Geometry: final body of the model. Coordinates: model frame, mm. A direction names the side the tool comes from. Give positions to 0.01 mm unless a question says otherwise; leave off trailing zeros. Order: outer loops, then holes, each group sorted by start corner. A loop starts at its lowest first (then second) coordinate and runs counter-clockwise, first axis right, second up. Notation, with made-up numbers: (26, 36.5) -> (45, 36.5) arc R34 cw to (45, 74.5) -> close; hole circle Ø6 at (-36.5, 16). An arc over 180 degrees is marked (long way). One line per question, with ' | ' between items. Start each with the question number.
(1) Set-up query: faces 1 (the face through (-11, 17.75, -5)), 2 (the face through (10.5, 0, 0)), 3 (the face through (-12, 0, 0)). Return all of +Z, -Z, +X, -X, +Y, -Y with unobstructed straight access to the full face (end or side cutting, diameter ignored); none if empty.
(2) First-contact query: pin 1 Ø2.5 at (x, z) = (-10.5, -1) entering from -Y; pin 2 Ø0.5 at (x, z) = (11.5, 5) entering from +Y; pin 3 Ø8 at (x, z) = (-3.5, 4) entering from +Y; pin 4 Ø1.2 at (x, y) = (11.5, 16) entering from +Z. Flat tips, straight axial feed; report the tip coordinate or a pass-through.
(3) Section D-D (y = 13.5). Return loops of the section in (x, z), then the cut area to 4 significant figures.
(4) Mould query, pull axis Z, two halves, no side actions, for faces 4 (the face through (11.49, 0.3, -9.76)), 5 (the face through (-11, -17.75, -5)), 6 (the face through (0, 0, 10.25)). Classes: +Z half, -Z half, draft (parallel to the pull), parting line (faces both ways), or undercut.
(5) Section B-B (z = -4). Return loops of the section in (x, y).
(6) Section C-C (x = -1.25). Return loops of the section in (y, z), then the cut area to 3 significant figures.
(7) Ray query, L1, parallel to Z at x = -1.5, y = 4; L2, parallel to X at y = 9.5, z = 7.5; L3, parallel to Z at x = 10.25, y = -3.5. Return the intervals inside material, ascending.
(8) Section A-A (z = -1.75). Return loops of the section in (x, y).
```python
from build123d import *

# Parameters (mm, degrees)
SKETCH2_W                       = 20.999999999999993
SKETCH2_H                       = 18.500000000000007
BOSS_EXTRUDE2_DEPTH             = 20.5
BOSS_EXTRUDE5_REACH             = 27.871
BOSS_EXTRUDE5_DIRECTION_2_REACH = 27.871
CUT_EXTRUDE1_DEPTH              = 34.81290434139014
CHAMFER1_SIZE                   = 1
CHAMFER1_OF_MIRROR1_SIZE        = 1


with BuildPart() as part:
    # Sketch2 → Boss-Extrude2 (new body)
    with BuildSketch(Plane(origin=(0, 0, 0), x_dir=(1, 0, 0), z_dir=(0, 1, 0))):
        Polygon((-11.999999999999991, -10.249999999999988), (12, -10.249999999999982), (11.999999999999998, 10.249999999999982), (-11.999999999999991, 10.249999999999979), align=None)
        Rectangle(SKETCH2_W, SKETCH2_H, mode=Mode.SUBTRACT)
    boss_extrude2 = extrude(amount=BOSS_EXTRUDE2_DEPTH)

    # Boss-Extrude5: up to this face of the body (flat: up to its plane)
    boss_extrude5_end = Plane(part.part.faces().sort_by_distance((12, 10.25, 0))[0])
    # Sketch4 → Boss-Extrude5 (add, up to the picked face)
    with BuildSketch(Plane(origin=(0, 0, 0), x_dir=(0, 0, -1), z_dir=(1, 0, 0)), mode=Mode.PRIVATE) as boss_extrude5_sk1:
        Polygon((-10.249999999999982, 20.5), (-9.249999999999988, 21.5), (-9.249999999999988, 20.5), align=None)
    boss_extrude5_tool1 = split(extrude(boss_extrude5_sk1.sketch, amount=BOSS_EXTRUDE5_REACH, mode=Mode.PRIVATE), bisect_by=boss_extrude5_end, keep=Keep.BOTH, mode=Mode.PRIVATE)
    # Sketch4 → Boss-Extrude5 (add, up to the picked face)
    with BuildSketch(Plane(origin=(0, 0, 0), x_dir=(0, 0, -1), z_dir=(1, 0, 0)), mode=Mode.PRIVATE) as boss_extrude5_sk2:
        Polygon((10.25, 20.500000000000004), (9.250000000000005, 21.500000000000004), (9.250000000000005, 20.500000000000004), align=None)
    boss_extrude5_tool2 = split(extrude(boss_extrude5_sk2.sketch, amount=BOSS_EXTRUDE5_REACH, mode=Mode.PRIVATE), bisect_by=boss_extrude5_end, keep=Keep.BOTH, mode=Mode.PRIVATE)
    boss_extrude5_1 = boss_extrude5_tool1.solids().sort_by(Axis((0, 20.833333, 9.583333), (1, 0, 0)))[0]
    add(boss_extrude5_1)
    boss_extrude5_2 = boss_extrude5_tool2.solids().sort_by(Axis((0, 20.833333, -9.583333), (1, 0, 0)))[0]
    add(boss_extrude5_2)
    boss_extrude5 = boss_extrude5_1 + boss_extrude5_2  # Boss-Extrude5 as one shape, for the pattern or mirror that repeats it

    # Boss-Extrude5 direction 2: up to this face of the body (flat: up to its plane)
    boss_extrude5_direction_2_end = Plane(part.part.faces().sort_by_distance((-12, 10.25, 0))[0])
    # Sketch4 → Boss-Extrude5 direction 2 (add, up to the picked face)
    with BuildSketch(Plane(origin=(0, 0, 0), x_dir=(0, 0, -1), z_dir=(1, 0, 0)), mode=Mode.PRIVATE) as boss_extrude5_direction_2_sk1:
        Polygon((-10.249999999999982, 20.5), (-9.249999999999988, 21.5), (-9.249999999999988, 20.5), align=None)
    boss_extrude5_direction_2_tool1 = split(extrude(boss_extrude5_direction_2_sk1.sketch, amount=-BOSS_EXTRUDE5_DIRECTION_2_REACH, mode=Mode.PRIVATE), bisect_by=boss_extrude5_direction_2_end, keep=Keep.BOTH, mode=Mode.PRIVATE)
    # Sketch4 → Boss-Extrude5 direction 2 (add, up to the picked face)
    with BuildSketch(Plane(origin=(0, 0, 0), x_dir=(0, 0, -1), z_dir=(1, 0, 0)), mode=Mode.PRIVATE) as boss_extrude5_direction_2_sk2:
        Polygon((10.25, 20.500000000000004), (9.250000000000005, 21.500000000000004), (9.250000000000005, 20.500000000000004), align=None)
    boss_extrude5_direction_2_tool2 = split(extrude(boss_extrude5_direction_2_sk2.sketch, amount=-BOSS_EXTRUDE5_DIRECTION_2_REACH, mode=Mode.PRIVATE), bisect_by=boss_extrude5_direction_2_end, keep=Keep.BOTH, mode=Mode.PRIVATE)
    boss_extrude5_direction_2_1 = boss_extrude5_direction_2_tool1.solids().sort_by(Axis((0, 20.833333, 9.583333), (-1, 0, 0)))[0]
    add(boss_extrude5_direction_2_1)
    boss_extrude5_direction_2_2 = boss_extrude5_direction_2_tool2.solids().sort_by(Axis((0, 20.833333, -9.583333), (-1, 0, 0)))[0]
    add(boss_extrude5_direction_2_2)
    boss_extrude5_direction_2 = boss_extrude5_direction_2_1 + boss_extrude5_direction_2_2  # Boss-Extrude5 direction 2 as one shape, for the pattern or mirror that repeats it

    # Sketch5 → Cut-Extrude1 (cut, through all)
    with BuildSketch(Plane(origin=(11.999999999999998, 0, -1.02e-15), x_dir=(0, 0, -1), z_dir=(1, 0, 0))):
        with BuildLine():
            Line((-6.9999999999999885, 17.750000000000004), (-2.9999999999999893, 17.750000000000004))
            ThreePointArc((-2.9999999999999893, 17.750000000000004), (-2.646446609406713, 17.603553390593277), (-2.4999999999999893, 17.25))
            Line((-2.4999999999999893, 17.25), (-2.4999999999999893, 15.75))
            ThreePointArc((-2.4999999999999893, 15.75), (-2.6464466094067154, 15.396446609406727), (-2.9999999999999893, 15.250000000000002))
            Line((-2.9999999999999893, 15.250000000000002), (-6.9999999999999885, 15.250000000000002))
            ThreePointArc((-6.9999999999999885, 15.250000000000002), (-7.353553390593261, 15.396446609406727), (-7.4999999999999885, 15.75))
            Line((-7.4999999999999885, 15.75), (-7.49999999999999, 17.25))
            ThreePointArc((-7.49999999999999, 17.25), (-7.353553390593265, 17.603553390593277), (-6.9999999999999885, 17.750000000000004))
        make_face()
        with BuildLine():
            Line((7.00000000000001, 17.750000000000004), (3.000000000000011, 17.750000000000004))
            ThreePointArc((3.000000000000011, 17.750000000000004), (2.646446609406735, 17.603553390593277), (2.500000000000011, 17.25))
            Line((2.500000000000011, 17.25), (2.500000000000011, 15.75))
            ThreePointArc((2.500000000000011, 15.75), (2.6464466094067376, 15.396446609406725), (3.000000000000012, 15.250000000000002))
            Line((3.000000000000012, 15.250000000000002), (7.0000000000000115, 15.250000000000004))
            ThreePointArc((7.0000000000000115, 15.250000000000004), (7.353553390593284, 15.39644660940673), (7.500000000000011, 15.750000000000004))
            Line((7.500000000000011, 15.750000000000004), (7.500000000000012, 17.250000000000004))
            ThreePointArc((7.500000000000012, 17.250000000000004), (7.3535533905932855, 17.603553390593277), (7.00000000000001, 17.750000000000004))
        make_face()
    cut_extrude1 = extrude(amount=-CUT_EXTRUDE1_DEPTH, mode=Mode.SUBTRACT)

    # Chamfer1
    chamfer1_edges = [part.edges().sort_by_distance(p)[0] for p in [
        (-11.999999999999991, 10.25, -10.249999999999979),
        (11.999999999999998, 10.25, -10.249999999999982),
        (12, 10.25, 10.249999999999982),
        (-11.999999999999991, 10.25, 10.249999999999988),
        (10.5, 10.25, -9.250000000000018),
        (-10.499999999999991, 10.25, -9.250000000000018),
        (-10.499999999999991, 10.25, 9.249999999999988),
        (10.5, 10.25, 9.249999999999988),
    ]]
    chamfer(chamfer1_edges, length=CHAMFER1_SIZE)


with BuildPart() as mirror1_1:
    # Mirror1: Boss-Extrude2, Boss-Extrude5, Boss-Extrude5 direction 2 across plane
    add(boss_extrude2.mirror(Plane.ZX))
    add(boss_extrude5.mirror(Plane.ZX))
    add(boss_extrude5_direction_2.mirror(Plane.ZX))

    # Mirror1 2: Cut-Extrude1 across plane
    add(cut_extrude1.mirror(Plane.ZX), mode=Mode.SUBTRACT)

    # Chamfer1 of Mirror1
    chamfer1_of_mirror1_edges = [mirror1_1.edges().sort_by_distance(p)[0] for p in [
        (-11.999999999999991, -10.25, -10.249999999999979),
        (11.999999999999998, -10.25, -10.249999999999982),
        (12, -10.25, 10.249999999999982),
        (-11.999999999999991, -10.25, 10.249999999999988),
        (10.5, -10.25, -9.250000000000018),
        (-10.499999999999991, -10.25, -9.250000000000018),
        (-10.499999999999991, -10.25, 9.249999999999988),
        (10.5, -10.25, 9.249999999999988),
    ]]
    chamfer(chamfer1_of_mirror1_edges, length=CHAMFER1_OF_MIRROR1_SIZE)


with BuildPart() as part_1:
    add(part.part)

    # Mirror1 united with what the copies touc: union Mirror1_1
    add(mirror1_1.part)


solid = part_1.part
```
Response:
1) face 1: +X, -X | face 2: +Y, -Y | face 3: +Z, -Z, -X, +Y, -Y
2) pin 1: stops at y = -20.5 | pin 2: stops at y = 20.5 | pin 3: passes through | pin 4: stops at z = 10.25
3) outline: (-12, -9.25) -> (-11, -10.25) -> (11, -10.25) -> (12, -9.25) -> (12, 9.25) -> (11, 10.25) -> (-11, 10.25) -> (-12, 9.25) -> close; hole (-10.5, -8.25) -> (-9.5, -9.25) -> (9.5, -9.25) -> (10.5, -8.25) -> (10.5, 8.25) -> (9.5, 9.25) -> (-9.5, 9.25) -> (-10.5, 8.25) -> close | area: 103.5 mm^2
4) face 4: -Z half | face 5: undercut | face 6: +Z half
5) outline: (-12, -20.5) -> (-10.5, -20.5) -> (-10.5, -17.75) -> (-12, -17.75) -> close; (-12, -15.25) -> (-10.5, -15.25) -> (-10.5, 15.25) -> (-12, 15.25) -> close; (-12, 17.75) -> (-10.5, 17.75) -> (-10.5, 20.5) -> (-12, 20.5) -> close; (10.5, -20.5) -> (12, -20.5) -> (12, -17.75) -> (10.5, -17.75) -> close; (10.5, -15.25) -> (12, -15.25) -> (12, 15.25) -> (10.5, 15.25) -> close; (10.5, 17.75) -> (12, 17.75) -> (12, 20.5) -> (10.5, 20.5) -> close
6) outline: (-21.5, -9.25) -> (-20.5, -10.25) -> (20.5, -10.25) -> (21.5, -9.25) -> close; (-21.5, 9.25) -> (21.5, 9.25) -> (20.5, 10.25) -> (-20.5, 10.25) -> close | area: 84.0 mm^2
7) L1: z = -10.25 to -9.25, 9.25 to 10.25 | L2: x = -12 to -10.5, 10.5 to 12 | L3: z = -10.25 to -8.5, 8.5 to 10.25
8) outline: (-12, -20.5) -> (-10.5, -20.5) -> (-10.5, 20.5) -> (-12, 20.5) -> close; (10.5, -20.5) -> (12, -20.5) -> (12, 20.5) -> (10.5, 20.5) -> close
